from build123d import *

# Parameters (mm, degrees)
F0_R     = 25.4758585114
F1_DEPTH = 101.6
F3_W     = 50.8
F3_H     = 50.8
F4_DEPTH = 57.658
F6_DEPTH = 57.658


# Not quite as in the source:
# - the program builds the solid bodies; features that only make, move or delete a surface that nothing else refers to are left out


with BuildPart() as f1:
    # F0 (on Front) → F1 (new body)
    with BuildSketch(Plane.XZ):
        Circle(F0_R)
    extrude(amount=F1_DEPTH)

    # F3 (on Front) → F4 (join)
    with BuildSketch(Plane.XZ):
        Rectangle(F3_W, F3_H)
    extrude(amount=-F4_DEPTH)

    # F5 (on Front) → F6 (join)
    with BuildSketch(Plane.XZ):
        Polygon((35.6535799801, 25.266315788), (0, 40.4261052608), (-35.6535799801, 25.266315788), align=None)
    extrude(amount=-F6_DEPTH)


solid = f1.part
Geometry check sheet. Reference: the model listing, model coordinates, mm. A direction names the side the tool comes from. Give positions to 0.01 mm unless a question says otherwise; leave off trailing zeros. Order: outer loops, then holes, each group sorted by start corner. A loop starts at its lowest first (then second) coordinate and runs counter-clockwise, first axis right, second up.
1. Sectioned sample at C-C (z = 0). Record the boundary of the cut face in (x, y), then the cut area to 3 significant figures.
Completed:
outline: (-25.48, -101.6) - (25.48, -101.6) - (25.48, 0) - (25.4, 0) - (25.4, 57.66) - (-25.4, 57.66) - (-25.4, 0) - (-25.48, 0) - close
area: 8,110 mm2
2. Sectioned sample at A-A (y = 16). Record the boundary of the cut face in (x, z).
Completed:
outline: (-35.65, 25.27) - (-25.4, 25.27) - (-25.4, -25.4) - (25.4, -25.4) - (25.4, 25.27) - (35.65, 25.27) - (0, 40.43) - close
3. Access from +Z, -Z, +X, -X, +Y, -Y to the whole of each face (thin tool, end or side, straight path). Record for faces 1 (the face through (-20, 0, -21)), 2 (the face through (0, 0, 26)), 3 (the face through (20, 0, -21)), 4 (the face through (23.53, -50.09, -9.76)), 5 (the face through (30, 28, 25.266)).
Completed:
face 1: -Z, -X, -Y
face 2: +Z, -Y
face 3: -Z, +X, -Y
face 4: -Y
face 5: -Z, +X, +Y, -Y
4. Depth check by flat-ended pin: pin 1 (4 mm diameter, centred on y = -80.5, z = 10, fed in from +X); pin 2 (3 mm diameter, centred on x = -28.5, y = 19.5, fed in from -Z); pin 3 (4 mm diameter, centred on x = 26.5, z = 29, fed in from -Y). Enter the tip coordinate at first touch or a pass-through.
Completed:
pin 1: stops at x = 24.19
pin 2: stops at z = 25.27
pin 3: stops at y = 0
5. Scan lines: line 1 (X direction, y = 28, z = 19); line 2 (Y direction, x = -21.5, z = 15.5); line 3 (Z direction, x = -23.5, y = 3.5). Record each from-to range of solid material in increasing order.
Completed:
line 1: x = -25.4 to 25.4
line 2: y = 0 to 57.66
line 3: z = -25.4 to 30.43
6. Sectioned sample at B-B (x = -6). Record the boundary of the cut face in (y, z).
Completed:
outline: (-101.6, -24.76) - (0, -24.76) - (0, -25.4) - (57.66, -25.4) - (57.66, 37.87) - (0, 37.87) - (0, 24.76) - (-101.6, 24.76) - close
7. Sectioned sample at D-D (y = -68). Record the boundary of the cut face in (x, z), then the cut area to 3 significant figures.
Completed:
outline: circle Ø50.95 at (0, 0)
area: 2,040 mm2
